The listing builds one solid part. Answer for the finished solid, in the listing's coordinates (mm). A direction names the side the tool comes from. Give positions to 0.01 mm unless a question says otherwise; leave off trailing zeros. One line per question, with ' | ' between items.
from build123d import *

# Parameters (mm, degrees)
SKETCH1_R           = 0.875
BOSS_EXTRUDE1_DEPTH = 6.35
SKETCH2_R           = 1.35
CUT_EXTRUDE1_DEPTH  = 12


with BuildPart() as part:
    # Sketch1 → Boss-Extrude1 (new body)
    with BuildSketch(Plane(origin=(0, 0, 0), x_dir=(1, 0, 0), z_dir=(0, 1, 0))):
        Polygon((0, 0), (0, 100), (0, 112), (18.25, 112), (18.25, 109.424759036), (21.549993184, 108.223659704), (21.549993186, 106.959378538), (18.25, 105.758279069), (18.25, 104.712379468), (21.549993194, 103.511280133), (21.549993196, 102.246998966), (18.25, 101.045899493), (18.25, 100), (21.549993184, 98.798900669), (21.549993186, 97.534619502), (18.25, 96.333520033), (18.25, 95.287620432), (21.549993194, 94.086521097), (21.549993196, 92.822239931), (18.25, 91.621140458), (18.25, 90.575240964), (21.549993204, 89.374141626), (21.549993207, 88.109860459), (18.25, 86.908760983), (18.25, 85.862861496), (21.549993214, 84.661762154), (21.549993217, 83.397480988), (18.25, 82.196381507), (18.25, 81.150481929), (21.549993224, 79.949382583), (21.549993227, 78.685101416), (18.25, 77.484001932), (18.25, 76.438102461), (21.549993234, 75.237003111), (21.549993237, 73.972721945), (18.25, 72.771622457), (18.25, 71.725722993), (21.549993244, 70.524623639), (21.549993247, 69.260342473), (18.25, 68.059242982), (18.25, 67.013343425), (21.549993254, 65.812244068), (21.549993257, 64.547962902), (18.25, 63.346863406), (18.25, 62.300963957), (21.549993265, 61.099864596), (21.549993267, 59.83558343), (18.25, 58.634483931), (18.25, 57.588584489), (21.549993275, 56.387485125), (21.549993277, 55.123203959), (18.25, 53.922104456), (18.25, 52.876204922), (21.549993285, 51.675105553), (21.549993288, 50.410824387), (18.25, 49.209724881), (18.25, 48.163825454), (21.549993295, 46.962726082), (21.549993298, 45.698444915), (18.25, 44.497345406), (18.25, 43.451445986), (21.549993305, 42.25034661), (21.549993308, 40.986065444), (18.25, 39.78496593), (18.25, 38.739066418), (21.549993315, 37.537967039), (21.549993318, 36.273685872), (18.25, 35.072586355), (18.25, 34.026686847), (21.549993325, 32.825587464), (21.549993328, 31.561306401), (18.25, 30.36020688), (18.25, 29.314307482), (21.549993336, 28.113208096), (21.549993338, 26.848926929), (18.25, 25.647827405), (18.25, 24.601927915), (21.549993346, 23.400828524), (21.549993348, 22.136547358), (18.25, 20.935447829), (18.25, 19.889548447), (21.549993356, 18.688449053), (21.549993359, 17.424167886), (18.25, 16.223068354), (18.25, 15.177168979), (21.549993366, 13.976069581), (21.549993369, 12.711788415), (18.25, 11.510688879), (18.25, 10.464789411), (21.549993376, 9.26369001), (21.549993379, 7.999408843), (18.25, 6.798309304), (18.25, 5), (23, 5), (23, 0), align=None)
        with Locations(Location((8.619246516, 95, 0), (0, 0, 270))):
            Circle(SKETCH1_R, mode=Mode.SUBTRACT)
        with Locations(Location((8.619246516, 65, 0), (0, 0, 270))):
            Circle(SKETCH1_R, mode=Mode.SUBTRACT)
        with Locations(Location((8.619246516, 35, 0), (0, 0, 270))):
            Circle(SKETCH1_R, mode=Mode.SUBTRACT)
        with Locations(Location((8.619246516, 5, 0), (0, 0, 270))):
            Circle(SKETCH1_R, mode=Mode.SUBTRACT)
    extrude(amount=BOSS_EXTRUDE1_DEPTH)

    # Sketch2 → Cut-Extrude1 (cut)
    with BuildSketch(Plane(origin=(0, 0, -112), x_dir=(-1, 0, 0), z_dir=(0, 0, -1))):
        with Locations((-13.625, 3.175)):
            Circle(SKETCH2_R)
        with Locations((-4.625, 3.175)):
            Circle(SKETCH2_R)
    extrude(amount=-CUT_EXTRUDE1_DEPTH, mode=Mode.SUBTRACT)


solid = part.part
Item 1: Flat-ended cylindrical pins translate along their axes: pin 1 (0.6 mm diameter, centred on y = 3.5, z = -65, fed in from +X); pin 2 (1.6 mm diameter, centred on x = 8.62, z = -95, fed in from -Y); pin 3 (0.8 mm diameter, centred on y = 2, z = -77, fed in from +X). Find the tip coordinate at first contact, or state that the pin passes through.
Answers below:
pin 1: x = 21.55 | pin 2: through | pin 3: x = 18.25
Item 2: Determine the mould class of faces 1 (the face through (5, 3, -100)), 2 (the face through (19.88, 3.13, -89.98)), 3 (the face through (9, 0, -57)) for opening direction X: pulls with the +X half, pulls with the -X half, needs draft (parallel to the pull), parting line crosses it, or undercut.
Answers below:
face 1: undercut | face 2: pulls with the +X half | face 3: needs draft
Item 3: A tool of negligible diameter and unlimited length cuts with its end or side. For faces 4 (the face through (23, 3, -3)), 5 (the face through (19.877, 3.131, -52.284)), 6 (the face through (14.62, 4.09, -106.08)), from which of +Z, -Z, +X, -X, +Y, -Y can it reach the whole face along a straight path? Write none if from no direction.
Answers below:
face 4: +Z, -Z, +X, +Y, -Y | face 5: +X, +Y, -Y | face 6: -Z
Item 4: Find section A-A (x = 20.25). Count the separate pieces of the cut face and the enclosed holes in it, then the cut area to 3 significant figures.
Answers below:
separate pieces: 23 | enclosed holes: 0 | area: 341 mm²
Item 5: Consider line 1 (X direction, y = 2.25, z = -65); line 2 (Z direction, x = 9, y = 2.75); line 3 (X direction, y = 2.5, z = -105). Determine where each line is inside the solid, lowest interval first. Write a range as [from, to].
Answers below:
line 1: [0, 7.74], [9.49, 21.55] | line 2: [-112, -95.79], [-94.21, -65.79], [-64.21, -35.79], [-34.21, -5.79], [-4.21, 0] | line 3: [0, 3.46], [5.79, 12.46], [14.79, 18.25]
